Model file for the job. Use its own axes, mm. A direction names the side the tool comes from. Round coordinates to 2 decimals unless told otherwise and drop trailing zeros. Loops run counter-clockwise (first coordinate to the right, second up) from the corner with the lowest first, then second, coordinate; pieces in that order, holes last. Notation, with made-up numbers: M 27,-24 L 41,-24 A13 ccw 41,-3 Z; hole C -13,0 d10. An arc over 180 degrees is marked long. Answer in a Markdown table with one row per item.
Autodesk Inventor part; units mm, degrees
ref_plane "Work Plane2" through (-22.5, 3, 0) normal (0, 1, 0) x (-1, 0, 0)
ref_plane "YZ Plane" through (0, 0, 0) normal (1, 0, 0) x (0, 1, 0)
ref_plane "XZ Plane" through (0, 0, 0) normal (0, 1, 0) x (-1, 0, 0)
sketch "Sketch15" plane through (0, 0, 0) normal (0, 1, 0) x (-1, 0, 0)
  line L0 (0, 0) -> (45, 0)
  line L1 (45, 0) -> (45, -20)
  line L2 (45, -20) -> (0, -20)
  line L3 (0, -20) -> (0, 0)
  dimension "d88" = 45
  dimension "d89" = 20
extrude "Extrusion11" add sketch "Sketch15" along normal blind 20
sketch "Sketch16" plane through (-45, 0, 0) normal (0, 0, 1) x (1, 0, 0)
  line L0 (45, 0) -> (45, 20)
  line L1 (0, 20) -> (45, 20)
  circle A0 centre (22.5, 10) radius 7
  dimension "d92" = 14
  dimension "d93" = 10
  dimension "d94" = 22.5
extrude "Extrusion12" add sketch "Sketch16" along normal blind 25
sketch "Sketch17" plane through (0, 0, 0) normal (1, 0, 0) x (0, 0, -1)
  line L0 (20, 0) -> (20, 20)
  line L1 (0, 0) -> (0, 20)
  line L2 (-25, 17) -> (-25, 3)
  line L3 (0, 3) -> (0, 17)
  line L4 (-25, 10) -> (20, 10) construction
  line L5 (0, 20) -> (20, 20)
  line L6 (20, 20) -> (20, 51)
  line L7 (0, 51) -> (0, 20)
  arc A0 (20, 51) -> (0, 51) centre (10, 51) ccw
  circle A1 centre (10, 51) radius 6.5 construction
  dimension "d98" = 41
  dimension "d99" = 13
extrude "Extrusion13" add sketch "Sketch17" against normal up to surface (45 mm away)
sketch "Sketch18" plane through (0, 0, -20) normal (0, 0, -1) x (-1, 0, 0)
  line L0 (0, 61) -> (45, 61)
  line L1 (9, 31) -> (36, 31)
  line L2 (36, 31) -> (36, 61)
  line L3 (36, 61) -> (9, 61)
  line L4 (9, 61) -> (9, 31)
  line L5 (45, 61) -> (45, 51)
  line L6 (0, 61) -> (0, 51)
  line L7 (0, 51) -> (45, 51)
  line L8 (14.6068, 31.9261) -> (20.6068, 31.9261)
  line L9 (20.6068, 31.9261) -> (20.6068, 53.9261)
  line L10 (20.6068, 53.9261) -> (14.6068, 53.9261)
  line L11 (14.6068, 53.9261) -> (14.6068, 31.9261)
  line L12 (20.6068, 25.659) -> (25.6068, 25.659)
  line L13 (25.6068, 25.659) -> (25.6068, 59.659)
  line L14 (25.6068, 59.659) -> (20.6068, 59.659)
  line L15 (20.6068, 59.659) -> (20.6068, 25.659)
  point P0 (40, 20)
  point P1 (0, 20)
  dimension "d105" = 30
  dimension "d106" = 9
  dimension "d107" = 9
  dimension "d116" = 20
  dimension "d117" = 6
  dimension "d118" = 22
  dimension "d119" = 5
  dimension "d120" = 34
  dimension "d121" = 10.3932
  dimension "d122" = 11.6068
extrude "Extrusion14" cut sketch "Sketch18" against normal through all contours L0 L2 L7 L13 L14 L15 L10 L11 L4 | L7 L11 L8 L15 L1 L4 | L2 L1 L13 L7 | L11 L10 L9 L7 | L7 L9 L8 L11 | L13 L1 L15 L9 L7 | L7 L9 L15 L14 L13
sketch "Sketch19" plane through (-36, 31, -20) normal (1, 0, 0) x (0, 0, -1)
  arc A0 (0, 20) -> (-20, 20) centre (-10, 20) ccw
  circle A1 centre (-10, 20) radius 6.5
  point P0 (-20, -31)
  point P1 (0, 22.9052)
  dimension "d110" = 13
extrude "Extrusion15" cut sketch "Sketch19" against normal blind 6
sketch "Sketch20" plane through (-9, 31, -20) normal (-1, 0, 0) x (0, 0, 1)
  arc A0 (20, 20) -> (0, 20) centre (10, 20) ccw
  circle A1 centre (10, 20) radius 6.5
  point P0 (20, -31)
  point P1 (0, 22.9052)
  dimension "d113" = 13
extrude "Extrusion16" cut sketch "Sketch20" against normal through all
sketch "Sketch21" plane through (0, 0, -20) normal (0, 0, -1) x (-1, 0, 0)
  line L0 (36, 31) -> (9, 31)
  line L1 (45, 0) -> (30, 0)
  line L2 (30, 0) -> (30, 31)
  line L3 (30, 31) -> (45, 31)
  line L4 (45, 31) -> (45, 0)
  line L5 (0, 0) -> (15, 0)
  line L6 (15, 0) -> (15, 31)
  line L7 (15, 31) -> (0, 31)
  line L8 (0, 31) -> (0, 0)
  line L9 (45, 0) -> (0, 0)
  line L10 (9, 31) -> (36, 31)
  line L11 (22.5, 31) -> (22.5, 0) construction
  point P0 (6, 19.5)
  point P1 (39, 19.5)
  dimension "d123" = 15
  dimension "d124" = 15
  dimension "d132" = 16.5
  dimension "d133" = 16.5
extrude "Extrusion17" [suppressed]
sketch "Sketch22" plane through (-45, 0, 0) normal (-1, 0, 0) x (0, 0, 1)
  line L0 (0, 0) -> (-20, 0)
  line L1 (-30, 23) -> (-20, 23)
  line L2 (-20, 23) -> (-20, 0)
  line L3 (-20, 0) -> (-30, 0)
  line L4 (-30, 0) -> (-30, 23)
  point P0 (-30, 0)
extrude "Extrusion18" [suppressed]
sketch "Sketch23" plane through (0, 51, -10) normal (1, 0, 0) x (0, 0, -1)
  line L0 (10, -43) -> (10, -20)
  line L1 (20, -43) -> (10, -43)
  line L2 (10, -43) -> (10, -20)
  line L3 (10, -20) -> (20, -20)
  line L4 (20, -20) -> (20, -43)
extrude "Extrusion19" [suppressed]
sketch "Sketch24" plane through (12, 43, -10) normal (1, 0, 0) x (0, 0, -1)
  line L0 (10, -20) -> (10, -43)
  line L1 (20, -20) -> (10, -20)
  line L2 (10, -20) -> (10, -31.5)
  line L3 (10, -31.5) -> (20, -31.5)
  line L4 (20, -31.5) -> (20, -20)
  point P0 (-10, -43)
revolve "Revolution1" [suppressed]
sketch "Sketch25" plane through (0, 0, -30) normal (0, 0, -1) x (-1, 0, 0)
  line L0 (15, 0) -> (-12, 0)
  line L1 (15, 0) -> (15, 23)
  line L2 (15, 23) -> (-12, 23)
  arc A0 (-12, 23) -> (-12, 0) centre (-12, 11.5) ccw
  point P0 (0, 0)
  point P1 (-3.6176, 11.5)
  point P2 (49.207, 11.5)
sketch "Sketch26" plane through (0, 0, -20) normal (0, 0, -1) x (-1, 0, 0)
  line L0 (0, 0) -> (0, 51)
  line L1 (45, 0) -> (0, 0)
  line L2 (45, 0) -> (45, 51)
  line L3 (-6.2428, 12) -> (58.3359, 12)
  point P0 (6, 12)
  point P1 (39, 12)
  dimension "d134" = 12
  dimension "d135" = 6
  dimension "d136" = 33
  dimension "d137" = 6
hole "Hole2" at (-39, 12, -20) direction (0, 0, 1) diameter 4 depth 6 tip angle 118
sketch "Sketch27" plane through (0, 0, 0) normal (1, 0, 0) x (0, 0, -1)
  line L0 (0, 10) -> (0, 14)
  line L1 (20, 14) -> (20, 10)
  line L2 (15, 16) -> (11, 16)
  line L3 (11, 16) -> (11, 8)
  line L4 (11, 8) -> (15, 8)
  line L5 (15, 8) -> (15, 16)
  line L6 (15, 12) -> (11, 12)
  line L7 (20, 14) -> (20, 10)
  line L8 (0, 0) -> (0, 51)
  line L9 (20, 14) -> (20, 10)
  line L10 (20, 31) -> (20, 51)
  line L11 (20, 0) -> (20, 51)
  line L12 (20, 0) -> (20, 51)
  line L13 (20, 51) -> (20, 31)
  line L14 (20, 14) -> (20, 10)
  line L15 (20, 12) -> (0, 12)
  dimension "d145" = 8
  dimension "d147" = 4
  dimension "d160" = 5
extrude "Extrusion20" cut sketch "Sketch27" against normal blind 12
sketch "Sketch28" plane through (0, 0, -20) normal (0, 0, -1) x (-1, 0, 0)
  line L0 (0, 0) -> (0, 51)
  line L1 (5, 12) -> (7.5, 12) construction
  line L2 (5, 10) -> (7.5, 10)
  line L3 (7.5, 14) -> (5, 14)
  arc A0 (5, 14) -> (5, 10) centre (5, 12) ccw
  arc A1 (7.5, 10) -> (7.5, 14) centre (7.5, 12) ccw
  point P0 (6.25, 12)
  dimension "d150" = 5
  dimension "d151" = 2.5
extrude "Extrusion21" cut sketch "Sketch28" against normal up to surface (9 mm away)
sketch "Sketch29" plane through (-45, 0, -20) normal (-1, 0, 0) x (0, 0, 1)
  line L0 (0, 0) -> (0, 51)
  line L1 (20, 0) -> (20, 43)
  line L2 (0, 10) -> (0, 14)
  line L3 (20, 14) -> (20, 10)
  line L4 (9, 16) -> (5, 16)
  line L5 (5, 16) -> (5, 8)
  line L6 (5, 8) -> (9, 8)
  line L7 (9, 8) -> (9, 16)
  line L8 (9, 12) -> (5, 12)
  line L9 (20, 14) -> (20, 10)
  line L10 (20, 12) -> (0, 12) construction
  line L11 (0, 10) -> (0, 14)
  dimension "d154" = 8
  dimension "d156" = 4
  dimension "d157" = 5
extrude "Extrusion22" cut sketch "Sketch29" against normal blind 12
ref_plane "Work Plane2" through (-22.5, 3, 0) normal (0, 1, 0) x (-1, 0, 0)
sketch "Sketch30" plane through (-22.5, 3, 0) normal (0, 1, 0) x (-1, 0, 0)
  line L0 (7, 25) -> (-7, 25)
  line L1 (-7, 0) -> (7, 0)
  point P0 (-22.5, 0)
  point P1 (0, 17)
  dimension "d161" = 8
hole "Hole3" at (-22.5, 3, 17) direction (0, 1, 0) diameter 3 depth 8 tip angle 118
equation "\"d106\" = d107"
equation "\"d124\" = d123"
properties part number "EndEffectorV2"
1. Saw through at C-C (x = -4). Write the cut outline in (y, z), and give its area (3 significant figures).
Verdict:
| item | result |
|---|---|
| outline | M 0,-20 L 10.27,-20 L 10.27,-15 L 8,-15 L 8,-11 L 16,-11 L 16,-15 L 13.73,-15 L 13.73,-20 L 51,-20 A10 ccw 51,0 L 0,0 Z; hole C 51,-10 d13 |
| area | 995 mm² |
2. Saw through at A-A (z = -10). Write the cut outline in (x, y), and give its area (3 significant figures).
Verdict:
| item | result |
|---|---|
| outline | M -45,0 L 0,0 L 0,44.5 L -9,44.5 L -9,31 L -36,31 L -36,44.5 L -42,44.5 L -42,57.5 L -36,57.5 L -36,61 L -45,61 Z; M -9,57.5 L 0,57.5 L 0,61 L -9,61 Z |
| area | 1,740 mm² |
3. Saw through at B-B (y = 56). Write the cut outline in (x, z).
Verdict:
| item | result |
|---|---|
| outline | M -45,-18.66 L -36,-18.66 L -36,-14.15 L -42,-14.15 L -42,-5.85 L -36,-5.85 L -36,-1.34 L -45,-1.34 Z; M -9,-18.66 L 0,-18.66 L 0,-14.15 L -9,-14.15 Z; M -9,-5.85 L 0,-5.85 L 0,-1.34 L -9,-1.34 Z |
4. Saw through at D-D (z = 6). Write the cut outline in (x, y).
Verdict:
| item | result |
|---|---|
| outline | C -22.5,10 d14 |
5. Pin check, flat tips, straight feed: pin 1 (10 mm diameter, centred on x = -26, y = 26.5, fed in from +Z); pin 2 (3 mm diameter, centred on x = -6, z = -16.5, fed in from +Y); pin 3 (4 mm diameter, centred on x = -22.5, z = 17, fed in from -Y). Stop position of each tip, or through.
Verdict:
| item | result |
|---|---|
| pin 1 | stops at z = 0 |
| pin 2 | stops at y = 59.66 |
| pin 3 | stops at y = 3 |
6. Tool access for faces 5 (the flat face through (-33, 12, -13)), 6 (the flat face through (-6, 14, -18)), 7 (the cylindrical face through (-4.563, 44.655, -11.409)): list every direction of +Z, -Z, +X, -X, +Y, -Y with a clear straight run to the whole face (end or side of a thin tool).
Verdict:
| item | result |
|---|---|
| face 5 | -X |
| face 6 | -Z |
| face 7 | +X |
7. Wall check: probe 1 along X at (y, z) = (12, -18); probe 2 along Y at (x, z) = (-3, -10); probe 3 along Z at (x, y) = (-9.5, 15). Give the ranges that are in metal, low to high.
Verdict:
| item | result |
|---|---|
| probe 1 | x = -45 to -41, -37 to -9.5, -3 to 0 |
| probe 2 | y = 0 to 44.5, 57.5 to 61 |
| probe 3 | z = -20 to -15, -11 to 0 |
8. Mould opens along Y. For faces 1 (the flat face through (-22, 0, -10)), 2 (the flat face through (-42, 51, -10)), 3 (the flat face through (-22, 19, -20)), 4 (the flat face through (-22, 31, -10)) say: +Y half, -Y half, draft (parallel to the pull), parting line (faces both ways), or undercut.
Verdict:
| item | result |
|---|---|
| face 1 | -Y half |
| face 2 | undercut |
| face 3 | draft |
| face 4 | +Y half |
